from build123d import *

# Parameters (mm, degrees)
EXTRUDE_1_DEPTH     = 10
EXTRUDE_START       = 30.8
SKETCH_4_W          = 54.5
SKETCH_4_H          = 20
EXTRUDE_2_DEPTH     = 2.4
SKETCH_5_R          = 2.25
CUT_EXTRUDE_1_DEPTH = 3.1
SKETCH_6_W          = 2
SKETCH_6_H          = 2.1
CUT_EXTRUDE_2_DEPTH = 3.1
SKETCH_8_R          = 6
EXTRUDE_3_DEPTH     = 1.9
EXTRUDE_3_DRAFT     = -30
SKETCH_9_R          = 2.5
EXTRUDE_4_DEPTH     = 4.1
SKETCH_10_R         = 1.25
CUT_EXTRUDE_3_DEPTH = 9
EXTRUDE_5_DEPTH     = 0.75
SKETCH_12_W         = 40
SKETCH_12_H         = 20
CUT_EXTRUDE_5_DEPTH = 2
FILLET_1_R          = 2
FILLET_2_R          = 0.5


with BuildPart() as part:
    # 草图3 → 凸台-拉伸1 (new, symmetric)
    with BuildSketch(Plane.XY):
        Polygon((-20, 0), (20, 0), (20, 35.1), (20, 38.8), (16, 38.8), (-13.8, 38.8), (-20, 38.8), (-20, 34.4), align=None)
    extrude(amount=EXTRUDE_1_DEPTH, both=True)

    # 草图4 → 凸台-拉伸2 (add)
    with BuildSketch(Plane(origin=(0, 0, 0), x_dir=(1, 0, 0), z_dir=(0, 1, 0)).offset(EXTRUDE_START)):
        Rectangle(SKETCH_4_W, SKETCH_4_H)
    extrude(amount=-EXTRUDE_2_DEPTH)

    # 草图5 → 切除-拉伸1 (cut)
    with BuildSketch(Plane(origin=(0, 30.8, 0), x_dir=(1, 0, 0), z_dir=(0, 1, 0))):
        with Locations(Location((-24.5, 5, 0), (0, 0, 270))):
            Circle(SKETCH_5_R)
        with Locations(Location((24.5, 5, 0), (0, 0, 270))):
            Circle(SKETCH_5_R)
        with Locations(Location((24.5, -5, 0), (0, 0, 270))):
            Circle(SKETCH_5_R)
        with Locations(Location((-24.5, -5, 0), (0, 0, 270))):
            Circle(SKETCH_5_R)
    extrude(amount=-CUT_EXTRUDE_1_DEPTH, mode=Mode.SUBTRACT)

    # 草图6 → 切除-拉伸2 (cut)
    with BuildSketch(Plane(origin=(0, 30.8, 0), x_dir=(1, 0, 0), z_dir=(0, 1, 0))):
        with Locations((-26.25, 5)):
            Rectangle(SKETCH_6_W, SKETCH_6_H)
        with Locations((26.25, 5)):
            Rectangle(SKETCH_6_W, SKETCH_6_H)
        with Locations((26.25, -5)):
            Rectangle(SKETCH_6_W, SKETCH_6_H)
        with Locations((-26.25, -5)):
            Rectangle(SKETCH_6_W, SKETCH_6_H)
    extrude(amount=-CUT_EXTRUDE_2_DEPTH, mode=Mode.SUBTRACT)


with BuildPart() as extrude_3_tool:
    # 草图8 → 凸台-拉伸3 (with draft: the straight prism first)
    with BuildSketch(Plane.XZ.offset(-40.7)):
        with Locations((-10.6, 0)):
            Circle(SKETCH_8_R)
    extrude(amount=EXTRUDE_3_DEPTH)
    # 凸台-拉伸3: the draft: its side faces are tilted about the plane it starts from
    extrude_3_sides = [extrude_3_tool.faces().sort_by_distance(p)[0] for p in [
        (-16.6, 39.75, 0),
    ]]
    draft(extrude_3_sides, Plane.XZ.offset(-40.7), EXTRUDE_3_DRAFT)


with BuildPart() as part_1:
    add(part.part)

    # 凸台-拉伸3: add extrude_3_tool
    add(extrude_3_tool.part)

    # 草图9 → 凸台-拉伸4 (add)
    with BuildSketch(Plane(origin=(0, 40.7, 0), x_dir=(1, 0, 0), z_dir=(0, 1, 0))):
        with Locations(Location((-10.6, 0, 0), (0, 0, 90))):
            Circle(SKETCH_9_R)
    extrude(amount=EXTRUDE_4_DEPTH)

    # 草图10 → 切除-拉伸3 (cut)
    with BuildSketch(Plane(origin=(0, 44.8, 0), x_dir=(1, 0, 0), z_dir=(0, 1, 0))):
        with Locations(Location((-10.6, 0, 0), (0, 0, 270))):
            Circle(SKETCH_10_R)
    extrude(amount=-CUT_EXTRUDE_3_DEPTH, mode=Mode.SUBTRACT)

    # 草图11 → 凸台-拉伸5 (add, symmetric)
    with BuildSketch(Plane.XY):
        Polygon((-20, 32.3), (-26, 30.8), (-20, 30.8), align=None)
        Polygon((20, 30.8), (20, 32.3), (26, 30.8), align=None)
    extrude(amount=EXTRUDE_5_DEPTH, both=True)

    # 草图12 → 切除-拉伸5 (cut)
    with BuildSketch(Plane(origin=(0, 38.8, 0), x_dir=(1, 0, 0), z_dir=(0, 1, 0))):
        Rectangle(SKETCH_12_W, SKETCH_12_H)
        with BuildLine():
            Line((-10.6, 9.3), (15, 9.3))
            Line((15, 9.3), (15, -9.3))
            Line((15, -9.3), (-10.6, -9.3))
            ThreePointArc((-10.6, -9.3), (-19.9, 0), (-10.6, 9.3))
        make_face(mode=Mode.SUBTRACT)
    extrude(amount=-CUT_EXTRUDE_5_DEPTH, mode=Mode.SUBTRACT)

    # 圆角1
    fillet_1_edges = [part_1.edges().sort_by_distance(p)[0] for p in [
        (20, 14.2, 10),
        (-20, 33.8, -10),
        (-20, 33.8, 10),
        (-20, 14.2, -10),
        (20, 33.8, -10),
        (-20, 14.2, 10),
        (20, 33.8, 10),
        (27.25, 29.6, 10),
        (-27.25, 29.6, -10),
        (27.25, 29.6, -10),
        (-27.25, 29.6, 10),
        (20, 14.2, -10),
    ]]
    fillet(fillet_1_edges, radius=FILLET_1_R)

    # 圆角2
    fillet_2_edges = [part_1.edges().sort_by_distance(p)[0] for p in [
        (-17.696965511, 38.8, 0),
        (-16.6, 40.7, 0),
    ]]
    fillet(fillet_2_edges, radius=FILLET_2_R)


solid = part_1.part
CAD build for the part. Positions are in the model's coordinates, mm. A direction names the side the tool comes from. Round coordinates to 2 decimals unless told otherwise and drop trailing zeros. Write each loop counter-clockwise with the first axis right and the second up, starting at its lowest first coordinate (ties: lowest second). Pieces come first, ordered by that corner, then holes. Notation, with made-up numbers: M -7,3 L 15,3 A17 ccw 15,25 Z; hole C 41,32 d3. An arc over 180 degrees is marked long. Put each result on its own line as item: value. Start each with the question number.
1) Saw through at A-A, the plane x = 24.5. Write the cut outline in (y, z) (3 decimals).
2) Saw through at D-D, the plane x = 0. Write the cut outline in (y, z).
3) Saw through at C-C, the plane y = 14.5. Write the cut outline in (x, z).
4) Pin check, flat tips, straight feed: pin 1 Ø10 at (x, z) = (21.5, -2.5) entering from +Y; pin 2 Ø1 at (x, y) = (-1, 38) entering from -Z; pin 3 Ø7 at (x, z) = (-24.5, -5) entering from -Y. Stop position of each tip, or through.
5) Drill centre lines: probe 1 along Z at (x, y) = (-24.5, 29.2); probe 2 along X at (y, z) = (43, 0); probe 3 along X at (y, z) = (22.5, 6.5). Where is each one in solid material? Low to high. Write a range as [from, to].
6) Pull direction Z, two halves, no side cores. Call faces 4 (the cylindrical face through (22.25, 29.62, 4.92)), 5 (the flat face through (24, 30.8, -2)), 6 (the flat face through (-22, 31, -0.75)), 7 (the cylindrical face through (-19.4, 33.76, 9.43)): pulls with the +Z half, pulls with the -Z half, needs draft (parallel to the pull), parting line crosses it, or undercut.
7) 3-axis set-ups, long thin cutter, end or side, ignore diameter. For faces 1 (the cylindrical face through (-19.4, 14, 9.43)), 2 (the flat face through (-20, 14, 0)), 3 (the flat face through (22, 31, -0.75)): which of +Z, -Z, +X, -X, +Y, -Y reach the whole face in a straight line?
Resolved:
1. outline: M 28.4,-10 L 30.8,-10 L 30.8,-7.25 L 28.4,-7.25 Z; M 28.4,-2.75 L 30.8,-2.75 L 30.8,-0.75 L 31.175,-0.75 L 31.175,0.75 L 30.8,0.75 L 30.8,2.75 L 28.4,2.75 Z; M 28.4,7.25 L 30.8,7.25 L 30.8,10 L 28.4,10 Z
2. outline: M 0,-10 L 36.8,-10 L 36.8,-9.3 L 38.8,-9.3 L 38.8,9.3 L 36.8,9.3 L 36.8,10 L 0,10 Z
3. outline: M -20,-8 A2 ccw -18,-10 L 18,-10 A2 ccw 20,-8 L 20,8 A2 ccw 18,10 L -18,10 A2 ccw -20,8 Z
4. pin 1: y = 36.8
4. pin 2: z = -9.3
4. pin 3: y = 28.4
5. probe 1: [-10, -7.25], [-2.75, 2.75], [7.25, 10]
5. probe 2: [-13.1, -11.85], [-9.35, -8.1]
5. probe 3: [-20, 20]
6. face 4: undercut
6. face 5: needs draft
6. face 6: pulls with the -Z half
6. face 7: pulls with the +Z half
7. face 1: +Z, -X, -Y
7. face 2: +Z, -Z, -X, -Y
7. face 3: -Z, +X, +Y
